from build123d import *

# Parameters (mm, degrees)
F0_R     = 31.75
F2_DEPTH = 12.7
F3_R     = 5.08
F4_DEPTH = 12.7
F5_DEPTH = 25.4
F6_ANGLE = 45
F7_R     = 2.54


with BuildPart() as f2:
    # F0 (on Top) → F2 (new body)
    with BuildSketch(Plane.XY):
        with BuildLine():
            ThreePointArc((37.2940384615, -7.7951712765), (37.8979739919, -3.9183628351), (38.1, 0))
            ThreePointArc((38.1, 0), (37.8979739919, 3.9183628351), (37.2940384615, 7.7951712765))
            ThreePointArc((37.2940384615, 7.7951712765), (26.9407683632, 26.9407683632), (7.7951712765, 37.2940384615))
            ThreePointArc((7.7951712765, 37.2940384615), (0, 38.1), (-7.7951712765, 37.2940384615))
            ThreePointArc((-7.7951712765, 37.2940384615), (-26.9407683632, -26.9407683632), (37.2940384615, -7.7951712765))
        make_face()
        Circle(F0_R, mode=Mode.SUBTRACT)
        with BuildLine():
            ThreePointArc((37.2940384615, 7.7951712765), (37.8979739919, 3.9183628351), (38.1, 0))
            ThreePointArc((38.1, 0), (37.8979739919, -3.9183628351), (37.2940384615, -7.7951712765))
            ThreePointArc((37.2940384615, -7.7951712765), (55.245, 0), (37.2940384615, 7.7951712765))
        make_face()
        with BuildLine():
            ThreePointArc((-7.7951712765, 37.2940384615), (0, 38.1), (7.7951712765, 37.2940384615))
            ThreePointArc((7.7951712765, 37.2940384615), (0, 55.245), (-7.7951712765, 37.2940384615))
        make_face()
        Circle(F0_R)
    extrude(amount=F2_DEPTH)

    # F3 (on face) → F4 (join)
    with BuildSketch(Plane.XY.offset(12.7)):
        with Locations((0, 20.32)):
            Circle(F3_R)
        with Locations((20.32, 0)):
            Circle(F3_R)
        with BuildLine():
            ThreePointArc((0, -24.13), (1.905, -22.225), (0, -20.32))
            ThreePointArc((0, -20.32), (-14.3684097937, -14.3684097937), (-20.32, 0))
            ThreePointArc((-20.32, 0), (-22.225, 1.905), (-24.13, 0))
            ThreePointArc((-24.13, 0), (-17.06248663, -17.06248663), (0, -24.13))
        make_face()
    extrude(amount=F4_DEPTH)

    # F0 (on Top) → F5 (join)
    with BuildSketch(Plane.XY):
        with BuildLine():
            ThreePointArc((37.2940384615, -7.7951712765), (37.8979739919, -3.9183628351), (38.1, 0))
            ThreePointArc((38.1, 0), (37.8979739919, 3.9183628351), (37.2940384615, 7.7951712765))
            ThreePointArc((37.2940384615, 7.7951712765), (26.9407683632, 26.9407683632), (7.7951712765, 37.2940384615))
            ThreePointArc((7.7951712765, 37.2940384615), (0, 38.1), (-7.7951712765, 37.2940384615))
            ThreePointArc((-7.7951712765, 37.2940384615), (-26.9407683632, -26.9407683632), (37.2940384615, -7.7951712765))
        make_face()
        Circle(F0_R, mode=Mode.SUBTRACT)
        with BuildLine():
            ThreePointArc((-7.7951712765, 37.2940384615), (0, 38.1), (7.7951712765, 37.2940384615))
            ThreePointArc((7.7951712765, 37.2940384615), (0, 55.245), (-7.7951712765, 37.2940384615))
        make_face()
        with BuildLine():
            ThreePointArc((37.2940384615, 7.7951712765), (37.8979739919, 3.9183628351), (38.1, 0))
            ThreePointArc((38.1, 0), (37.8979739919, -3.9183628351), (37.2940384615, -7.7951712765))
            ThreePointArc((37.2940384615, -7.7951712765), (55.245, 0), (37.2940384615, 7.7951712765))
        make_face()
    extrude(amount=F5_DEPTH)


with BuildPart() as f2_1:
    # F6: moved
    add(f2.part.rotate(Axis((0, 0, 29.6926), (0, 0, 1)), F6_ANGLE))

    # F7
    f7_edges = [f2_1.edges().sort_by_distance(p)[0] for p in [
        (-20.858849, 31.882886, 12.7),
        (-31.882886, 20.858849, 12.7),
        (31.882886, 20.858849, 12.7),
        (20.858849, 31.882886, 12.7),
    ]]
    fillet(f7_edges, radius=F7_R)


solid = f2_1.part
For this review, take the finished solid that the model builds, in its own axes (mm). A direction names the side the tool comes from. Round coordinates to 2 decimals unless told otherwise and drop trailing zeros. Loops run counter-clockwise (first coordinate to the right, second up) from the corner with the lowest first, then second, coordinate; pieces in that order, holes last. Notation, with made-up numbers: (-25, -5.5) - (23, -5.5) arc R18 cw to (23, 18.5) - close; hole circle Ø3 at (-17.75, 15). An arc over 180 degrees is marked (long way). One line per item, written item: value. Start each with the question number.
Item 1: Take a section at B-B (x = 0). Give the boundary of the cut face in (y, z).
Item 2: Take a section at A-A (y = 0). Give the boundary of the cut face in (x, z).
Item 3: Take a section at C-C (y = -9). Give the boundary of the cut face in (x, z), plus the area to 3 significant figures.
Item 4: The part is to be moulded in two halves that separate along X. For faces 1 (the cylindrical face through (-1.098, -38.084, 12.522)), 2 (the flat face through (6, 5, 0)), 3 (the cylindrical face through (-0.27, -24.13, 18.96)), say which applies: +X half, -X half, draft (parallel to the pull), parting line (faces both ways), or undercut.
Item 5: For L1, parallel to Y at x = 14.5, z = 14.25; L2, parallel to Y at x = 18, z = 12.75; L3, parallel to X at y = 0, z = 19.75, list the stretches that pass through material, from the lowest coordinate up.
Item 6: Take a section at D-D (y = 13.5). Give the boundary of the cut face in (x, z).
Item 7: For faces 4 (the flat face through (-5, 32, 25.4)), 5 (the cylindrical face through (17.05, -26.784, 18.961)), list the 3-axis set-ups (+Z, -Z, +X, -X, +Y, -Y) from which the entire face can be reached by the end or side of a thin tool; tool diameter is ignored.
Item 8: Clearance check with flat-ended pins moving along their axes: pin 1 Ø1.5 at (y, z) = (-8, 19) entering from -X; pin 2 Ø2 at (y, z) = (-5, 13) entering from +X; pin 3 Ø3 at (y, z) = (-29, 9) entering from -X. State where each tip first meets the part, or that it passes through.
Answer below:
1. outline: (-38.1, 0) - (38.1, 0) - (38.1, 25.4) - (31.75, 25.4) - (31.75, 12.7) - (-20.32, 12.7) - (-20.32, 25.4) - (-24.13, 25.4) - (-24.13, 12.7) - (-31.75, 12.7) - (-31.75, 25.4) - (-38.1, 25.4) - close
2. outline: (-38.1, 0) - (38.1, 0) - (38.1, 25.4) - (31.75, 25.4) - (31.75, 12.7) - (-31.75, 12.7) - (-31.75, 25.4) - (-38.1, 25.4) - close
3. outline: (-37.02, 0) - (37.02, 0) - (37.02, 25.4) - (30.45, 25.4) - (30.45, 12.7) - (-30.45, 12.7) - (-30.45, 25.4) - (-37.02, 25.4) - close
3. area: 1,110 mm2
4. face 1: parting line
4. face 2: draft
4. face 3: undercut
5. L1: y = -35.23 to -28.25, -19.29 to -14.25, 9.29 to 19.45, 28.25 to 35.23
5. L2: y = -33.58 to -26.15, 10.82 to 17.92, 26.15 to 33.59
5. L3: x = -38.1 to -31.75, 31.75 to 38.1
6. outline: (-35.63, 0) - (35.63, 0) - (35.63, 25.4) - (28.74, 25.4) - (28.74, 12.7) - (19.37, 12.7) - (19.37, 25.4) - (9.36, 25.4) - (9.36, 12.7) - (-9.36, 12.7) - (-9.36, 25.4) - (-19.37, 25.4) - (-19.37, 12.7) - (-28.74, 12.7) - (-28.74, 25.4) - (-35.63, 25.4) - close
7. face 4: +Z, +X, -X, +Y, -Y
7. face 5: +Z
8. pin 1: stops at x = -37.4
8. pin 2: stops at x = 37.89
8. pin 3: stops at x = -26.37
